Verification items for the finished model (mm, model axes). A direction names the side the tool comes from. Round coordinates to 2 decimals unless told otherwise and drop trailing zeros. Write each loop counter-clockwise with the first axis right and the second up, starting at its lowest first coordinate (ties: lowest second). Pieces come first, ordered by that corner, then holes.
from build123d import *

# Parameters (mm, degrees)
F0_W      = 101.6
F0_H      = 101.6
F1_DEPTH  = 25.4
F2_W      = 88.9
F2_H      = 88.9
F3_DEPTH  = 25.4
F4_W      = 76.2
F4_H      = 76.2
F5_DEPTH  = 25.4
F6_W      = 63.5
F6_H      = 63.5
F7_DEPTH  = 19.05
F8_W      = 50.8
F8_H      = 50.8
F9_DEPTH  = 19.05
F10_W     = 38.1
F10_H     = 38.1
F11_DEPTH = 19.05


with BuildPart() as f1:
    # F0 (on Top) → F1 (new body)
    with BuildSketch(Plane.XY):
        with Locations((50.8, 50.8)):
            Rectangle(F0_W, F0_H)
        with Locations((-50.8, 50.8)):
            Rectangle(F0_W, F0_H)
        with Locations((-50.8, -50.8)):
            Rectangle(F0_W, F0_H)
        with Locations((50.8, -50.8)):
            Rectangle(F0_W, F0_H)
    extrude(amount=F1_DEPTH)

    # F2 (on face) → F3 (join)
    with BuildSketch(Plane.XY.offset(25.4)):
        with Locations((44.45, 44.45)):
            Rectangle(F2_W, F2_H)
        with Locations((44.45, -44.45)):
            Rectangle(F2_W, F2_H)
        with Locations((-44.45, -44.45)):
            Rectangle(F2_W, F2_H)
        with Locations((-44.45, 44.45)):
            Rectangle(F2_W, F2_H)
    extrude(amount=F3_DEPTH)

    # F4 (on face) → F5 (join)
    with BuildSketch(Plane.XY.offset(50.8)):
        with Locations((38.1, 38.1)):
            Rectangle(F4_W, F4_H)
        with Locations((38.1, -38.1)):
            Rectangle(F4_W, F4_H)
        with Locations((-38.1, -38.1)):
            Rectangle(F4_W, F4_H)
        with Locations((-38.1, 38.1)):
            Rectangle(F4_W, F4_H)
    extrude(amount=F5_DEPTH)

    # F6 (on face) → F7 (join)
    with BuildSketch(Plane.XY.offset(76.2)):
        with Locations((31.75, -31.75)):
            Rectangle(F6_W, F6_H)
        with Locations((-31.75, -31.75)):
            Rectangle(F6_W, F6_H)
        with Locations((31.75, 31.75)):
            Rectangle(F6_W, F6_H)
        with Locations((-31.75, 31.75)):
            Rectangle(F6_W, F6_H)
    extrude(amount=F7_DEPTH)

    # F8 (on face) → F9 (join)
    with BuildSketch(Plane.XY.offset(95.25)):
        with Locations((25.4, 25.4)):
            Rectangle(F8_W, F8_H)
        with Locations((25.4, -25.4)):
            Rectangle(F8_W, F8_H)
        with Locations((-25.4, -25.4)):
            Rectangle(F8_W, F8_H)
        with Locations((-25.4, 25.4)):
            Rectangle(F8_W, F8_H)
    extrude(amount=F9_DEPTH)

    # F10 (on face) → F11 (join)
    with BuildSketch(Plane.XY.offset(114.3)):
        with Locations((-19.05, -19.05)):
            Rectangle(F10_W, F10_H)
        with Locations((19.05, -19.05)):
            Rectangle(F10_W, F10_H)
        with Locations((19.05, 19.05)):
            Rectangle(F10_W, F10_H)
        with Locations((-19.05, 19.05)):
            Rectangle(F10_W, F10_H)
    extrude(amount=F11_DEPTH)


solid = f1.part
Q1. Sectioned sample at D-D (y = 57). Enter the section's corners in (x, z).
Recorded:
outline: (-101.6, 0) - (101.6, 0) - (101.6, 25.4) - (88.9, 25.4) - (88.9, 50.8) - (76.2, 50.8) - (76.2, 76.2) - (63.5, 76.2) - (63.5, 95.25) - (-63.5, 95.25) - (-63.5, 76.2) - (-76.2, 76.2) - (-76.2, 50.8) - (-88.9, 50.8) - (-88.9, 25.4) - (-101.6, 25.4) - close
Q2. Material ranges on line 1 along Z through (x, y) = (-2, -88.5); line 2 along Z through (x, y) = (43, -32); line 3 along Y through (x, z) = (72, 30), recorded low to high.
Recorded:
line 1: z = 0 to 50.8
line 2: z = 0 to 114.3
line 3: y = -88.9 to 88.9
Q3. Sectioned sample at A-A (y = -68). Enter the section's corners in (x, z), plus the area to 3 significant figures.
Recorded:
outline: (-101.6, 0) - (101.6, 0) - (101.6, 25.4) - (88.9, 25.4) - (88.9, 50.8) - (76.2, 50.8) - (76.2, 76.2) - (-76.2, 76.2) - (-76.2, 50.8) - (-88.9, 50.8) - (-88.9, 25.4) - (-101.6, 25.4) - close
area: 13,500 mm2
Q4. Depth check by flat-ended pin: P1, Ø9.5, axis at y = 10, z = 108, coming from the -X side; P2, Ø5.5, axis at y = -3, z = 126.5, coming from the -X side; P3, Ø10, axis at x = 53.5, z = 116.5, coming from the -Y side. Enter the tip coordinate at first touch or a pass-through.
Recorded:
P1: stops at x = -50.8
P2: stops at x = -38.1
P3: stops at y = -50.8
Q5. Tool access check on faces 1 (the flat face through (50.8, -1, 105)), 2 (the flat face through (-1, -63.5, 86)), 3 (the flat face through (-76.2, 1, 63)), 4 (the flat face through (1, 63.5, 86)), 5 (the flat face through (-1, 1, 133.35)). Record the directions out of +Z, -Z, +X, -X, +Y, -Y that give a thin tool (end or side, any length) a straight path to the whole face; none if there is none.
Recorded:
face 1: +Z, +X, +Y, -Y
face 2: +Z, +X, -X, -Y
face 3: +Z, -X, +Y, -Y
face 4: +Z, +X, -X, +Y
face 5: +Z, +X, -X, +Y, -Y
Q6. Sectioned sample at C-C (z = 80.5). Enter the section's corners in (x, y), plus the area to 3 significant figures.
Recorded:
outline: (-63.5, -63.5) - (63.5, -63.5) - (63.5, 63.5) - (-63.5, 63.5) - close
area: 16,100 mm2
